For this review, take the finished solid that the model builds, in its own axes (mm). A direction names the side the tool comes from. Round coordinates to 2 decimals unless told otherwise and drop trailing zeros. Order: outer loops, then holes, each group sorted by start corner. A loop starts at its lowest first (then second) coordinate and runs counter-clockwise, first axis right, second up. Notation, with made-up numbers: (78.5, -26) -> (112.5, -26) arc R15 ccw to (112.5, -16) -> close; hole circle Ø6 at (73.5, 44.25). An arc over 180 degrees is marked (long way). Use a Markdown table: item, result. Add a question column.
1) Clearance check with flat-ended pins moving along their axes: P1, Ø1.5, axis at x = -17, z = 34.5, coming from the -Y side; P2, Ø5, axis at x = 11, y = 7.5, coming from the +Z side; P3, Ø3, axis at y = 7.5, z = -19, coming from the +X side; P4, Ø1.5, axis at x = 5.5, y = 7, coming from the +Z side. State where each tip first meets the part, or that it passes through.
2) Consider section A-A (z = 0). State the section outline as (x, y) points, plus the area to 3 significant figures.
3) Consider section B-B (x = 0). State the section outline as (y, z) points.
4) Machinability: for faces 1 (the face through (40, 9.59, 7)), 2 (the face through (-39.05, 0.49, -8.67)), 3 (the face through (38.668, 9.083, -5.077)), which of the approach directions +Z, -Z, +X, -X, +Y, -Y give a long, thin tool a straight path to every point of the face, cutting with its end or side? Answer none if there is none.
5) Wall thickness on line 1 along X through (y, z) = (9.35, 0); line 2 along X through (y, z) = (4, 8); line 3 along Z through (x, y) = (19, 8.75): over which ranges is each line inside the solid? List them lowest first. Write a range as [from, to].
6) Consider section D-D (x = -32). State the section outline as (y, z) points.
7) Draft analysis for pull direction X (two halves, no side actions). For faces 4 (the face through (-43.028, 4.728, 22.38)), 5 (the face through (-38.3, 1, 8.7)), 6 (the face through (-23, 9.59, 20)), state which applies: pulls with the +X half, pulls with the -X half, needs draft (parallel to the pull), parting line crosses it, or undercut.
8) Consider section C-C (y = 3.75). State the section outline as (x, z) points.
```python
from build123d import *

# Parameters (mm, degrees)
SKETCH1_R           = 48.5
SKETCH1_R_2         = 30
BOSS_EXTRUDE1_DEPTH = 9.59
SKETCH2_R           = 40
SKETCH2_R_2         = 39
CUT_EXTRUDE1_DEPTH  = 1
CUT_EXTRUDE2_START  = -1
SKETCH3_R           = 40
SKETCH3_R_2         = 39
CUT_EXTRUDE2_DEPTH  = 1


with BuildPart() as part:
    # Sketch1 → Boss-Extrude1 (new body)
    with BuildSketch(Plane(origin=(0, 0, 0), x_dir=(1, 0, 0), z_dir=(0, 1, 0))):
        with Locations(Location((0, 0, 0), (0, 0, 270))):
            Circle(SKETCH1_R)
        with Locations(Location((0, 0, 0), (0, 0, 270))):
            Circle(SKETCH1_R_2, mode=Mode.SUBTRACT)
    extrude(amount=BOSS_EXTRUDE1_DEPTH)

    # Sketch2 → Cut-Extrude1 (cut)
    with BuildSketch(Plane(origin=(0, 0, 0), x_dir=(1, 0, 0), z_dir=(0, 1, 0))):
        with Locations(Location((0, 0, 0), (0, 0, 270))):
            Circle(SKETCH2_R)
        with Locations(Location((0, 0, 0), (0, 0, 270))):
            Circle(SKETCH2_R_2, mode=Mode.SUBTRACT)
    extrude(amount=CUT_EXTRUDE1_DEPTH, mode=Mode.SUBTRACT)

    # Sketch3 → Cut-Extrude2 (cut)
    with BuildSketch(Plane(origin=(0, 9.59, 0), x_dir=(1, 0, 0), z_dir=(0, 1, 0)).offset(CUT_EXTRUDE2_START)):
        with Locations(Location((0, 0, 0), (0, 0, 270))):
            Circle(SKETCH3_R)
        with Locations(Location((0, 0, 0), (0, 0, 270))):
            Circle(SKETCH3_R_2, mode=Mode.SUBTRACT)
    extrude(amount=CUT_EXTRUDE2_DEPTH, mode=Mode.SUBTRACT)


solid = part.part
```
Results list:
| question | item | result |
|---|---|---|
| 1 | P1 | y = 0 |
| 1 | P2 | z = 47.75 |
| 1 | P3 | x = 45.23 |
| 1 | P4 | z = 48.27 |
| 2 | outline | (-48.5, 0) -> (-40, 0) -> (-40, 1) -> (-39, 1) -> (-39, 0) -> (-30, 0) -> (-30, 9.59) -> (-39, 9.59) -> (-39, 8.59) -> (-40, 8.59) -> (-40, 9.59) -> (-48.5, 9.59) -> close; (30, 0) -> (39, 0) -> (39, 1) -> (40, 1) -> (40, 0) -> (48.5, 0) -> (48.5, 9.59) -> (40, 9.59) -> (40, 8.59) -> (39, 8.59) -> (39, 9.59) -> (30, 9.59) -> close |
| 2 | area | 351 mm2 |
| 3 | outline | (0, -48.5) -> (9.59, -48.5) -> (9.59, -40) -> (8.59, -40) -> (8.59, -39) -> (9.59, -39) -> (9.59, -30) -> (0, -30) -> (0, -39) -> (1, -39) -> (1, -40) -> (0, -40) -> close; (0, 30) -> (9.59, 30) -> (9.59, 39) -> (8.59, 39) -> (8.59, 40) -> (9.59, 40) -> (9.59, 48.5) -> (0, 48.5) -> (0, 40) -> (1, 40) -> (1, 39) -> (0, 39) -> close |
| 4 | face 1 | +Z, -Z, +X, -X, +Y |
| 4 | face 2 | -Y |
| 4 | face 3 | +Y |
| 5 | line 1 | [-48.5, -40], [-39, -30], [30, 39], [40, 48.5] |
| 5 | line 2 | [-47.84, -28.91], [28.91, 47.84] |
| 5 | line 3 | [-44.62, -35.2], [-34.06, -23.22], [23.22, 34.06], [35.2, 44.62] |
| 6 | outline | (0, -36.45) -> (9.59, -36.45) -> (9.59, -24) -> (8.59, -24) -> (8.59, -22.29) -> (9.59, -22.29) -> (9.59, 22.29) -> (8.59, 22.29) -> (8.59, 24) -> (9.59, 24) -> (9.59, 36.45) -> (0, 36.45) -> (0, 24) -> (1, 24) -> (1, 22.29) -> (0, 22.29) -> (0, -22.29) -> (1, -22.29) -> (1, -24) -> (0, -24) -> close |
| 7 | face 4 | parting line crosses it |
| 7 | face 5 | undercut |
| 7 | face 6 | needs draft |
| 8 | outline | circle Ø97 at (0, 0); hole circle Ø60 at (0, 0) |
